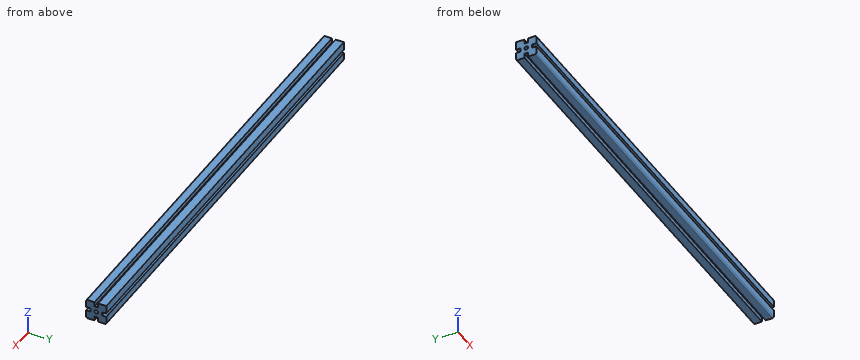
```python
from build123d import *

# Parameters (mm, degrees)
ESQUISSE1_R        = 4
BOSS_EXTRU_1_DEPTH = 978
CONG_1_R           = 3


with BuildPart() as part:
    # Esquisse1 → Boss.-Extru.1 (new body)
    with BuildSketch(Plane(origin=(1000, 0, 0), x_dir=(0, 0, -1), z_dir=(1, 0, 0))):
        Polygon((22.5, -4), (12.5, -4), (12.5, 4), (22.5, 4), (22.5, 22.5), (4, 22.5), (4, 12.5), (-4, 12.5), (-4, 22.5), (-22.5, 22.5), (-22.5, 4), (-12.5, 4), (-12.5, -4), (-22.5, -4), (-22.5, -22.5), (-4, -22.5), (-4, -12.5), (4, -12.5), (4, -22.5), (22.5, -22.5), align=None)
        Circle(ESQUISSE1_R, mode=Mode.SUBTRACT)
    extrude(amount=-BOSS_EXTRU_1_DEPTH)

    # Congé1
    cong_1_edges = [part.edges().sort_by_distance(p)[0] for p in [
        (511, -22.5, -22.5),
        (511, -12.5, -4),
        (511, -22.5, 22.5),
        (511, 22.5, -22.5),
    ]]
    fillet(cong_1_edges, radius=CONG_1_R)


solid = part.part
```
Geometry check sheet. Reference: the model listing, model coordinates, mm. Round coordinates to 2 decimals unless told otherwise and drop trailing zeros. Order: outer loops, then holes, each group sorted by start corner. A loop starts at its lowest first (then second) coordinate and runs counter-clockwise, first axis right, second up. Notation, with made-up numbers: (82, 78) - (101, 78) arc R27 ccw to (101, 100) - close; hole circle Ø5 at (22.25, -33.75). An arc over 180 degrees is marked (long way). Use a Markdown table: item, result. Add a question column.
(1) Material ranges on line 1 along Z through (x, y) = (652, 16); line 2 along Y through (x, z) = (326.5, 0); line 3 along Y through (x, z) = (865, -20), recorded low to high. Write a range as [from, to].
(2) Depth check by flat-ended pin: pin 1 (4 mm diameter, centred on x = 494, y = -0.5, fed in from -Z); pin 2 (10.5 mm diameter, centred on y = 0, z = 0, fed in from +X); pin 3 (2.5 mm diameter, centred on x = 552.5, y = 1, fed in from +Z); pin 4 (2.5 mm diameter, centred on x = 622, z = 0.5, fed in from -Y). Enter the tip coordinate at first touch or a pass-through.
(3) Sectioned sample at A-A, the plane x = 287. Enter the section's corners in (y, z), and give its area (3 significant figures).
Answers below:
| question | item | result |
|---|---|---|
| 1 | line 1 | [-22.5, -4], [4, 22.5] |
| 1 | line 2 | [-12.5, -4], [4, 12.5] |
| 1 | line 3 | [-22.46, -4], [4, 22.46] |
| 2 | pin 1 | z = -12.5 |
| 2 | pin 2 | x = 1000 |
| 2 | pin 3 | z = 12.5 |
| 2 | pin 4 | y = -12.5 |
| 3 | outline | (-22.5, -19.5) arc R3 ccw to (-19.5, -22.5) - (-4, -22.5) - (-4, -12.5) - (4, -12.5) - (4, -22.5) - (19.5, -22.5) arc R3 ccw to (22.5, -19.5) - (22.5, -4) - (12.5, -4) - (12.5, 4) - (22.5, 4) - (22.5, 22.5) - (4, 22.5) - (4, 12.5) - (-4, 12.5) - (-4, 22.5) - (-19.5, 22.5) arc R3 ccw to (-22.5, 19.5) - (-22.5, 4) - (-12.5, 4) - (-12.5, -1) arc R3 cw to (-15.5, -4) - (-22.5, -4) - close; hole circle Ø8 at (0, 0) |
| 3 | area | 1,650 mm² |
